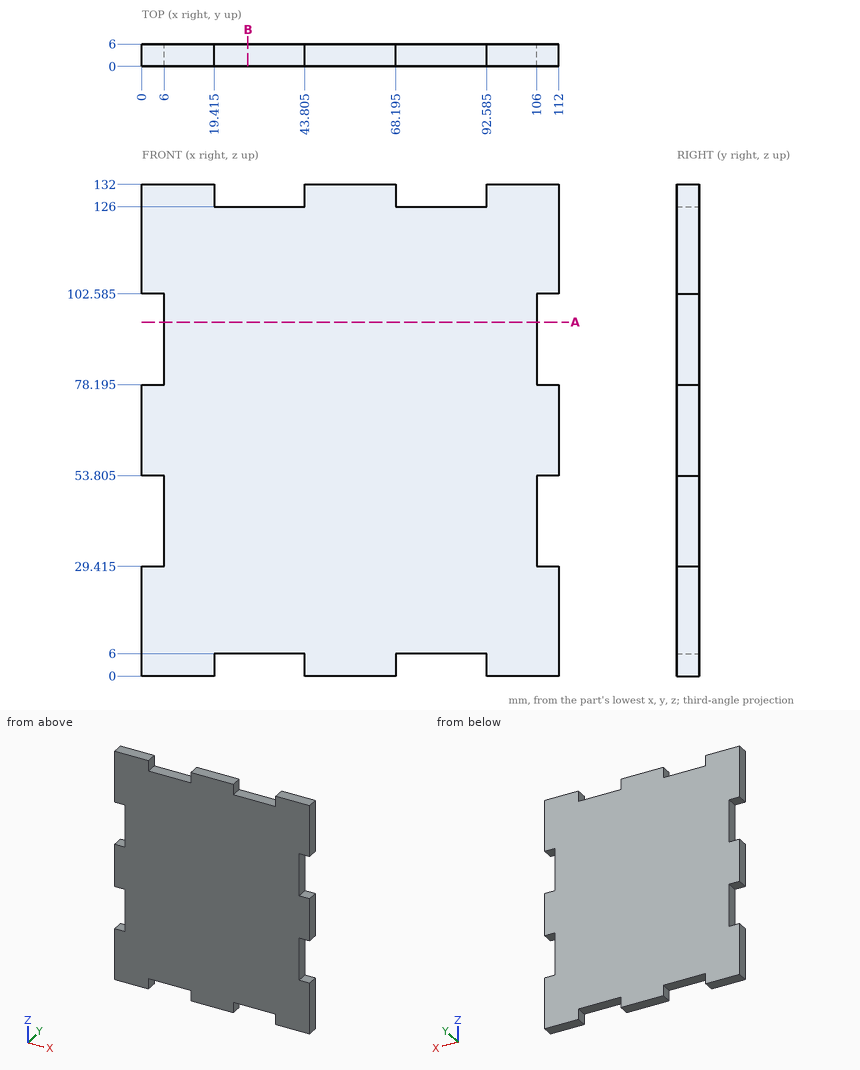
Geometry: see drawing. Coordinates: mm, zero at the bounding-box minimum. Coordinates: 2 decimals unless noted, no trailing zeros. Order: outer loops, then holes, each group sorted by start corner. A loop starts at its lowest first (then second) coordinate and runs counter-clockwise, first axis right, second up. Notation, with made-up numbers: (-14, -18) - (10, -18) arc R30 cw to (10, 11) - close; hole circle Ø5 at (61, -24.75). An arc over 180 degrees is marked (long way). Return JSON: item names as keys, results as strings.
Q1. First-contact query: pin 1 (1.5 mm diameter, centred on x = 91.5, y = 2.5, fed in from -Z); pin 2 (3 mm diameter, centred on y = 2, z = 38, fed in from +X); pin 3 (8 mm diameter, centred on x = 86, z = 17.5, fed in from -Y). Flat tips, straight axial feed; report the tip coordinate or a pass-through.
The answers:
{"pin 1": "stops at z = 6", "pin 2": "stops at x = 106", "pin 3": "stops at y = 0"}
Q2. Cut plane A-A (z = 95). Return loops of the section in (x, y).
The answers:
{"outline": "(6, 0) - (106, 0) - (106, 6) - (6, 6) - close"}
Q3. Cut plane B-B (x = 28.5). Return loops of the section in (y, z), then the cut area to 3 significant figures.
The answers:
{"outline": "(0, 6) - (6, 6) - (6, 126) - (0, 126) - close", "area": "720 mm2"}
Q4. Ray query, probe 1 along Z at (x, y) = (78.5, 0.4); probe 2 along X at (y, z) = (0.4, 90). Return the intervals inside material, ascending.
The answers:
{"probe 1": "z = 6 to 126", "probe 2": "x = 6 to 106"}
